Model file for the job. Use its own axes, mm. A direction names the side the tool comes from. Round coordinates to 2 decimals unless told otherwise and drop trailing zeros. Loops run counter-clockwise (first coordinate to the right, second up) from the corner with the lowest first, then second, coordinate; pieces in that order, holes last. Notation, with made-up numbers: M 62,-6 L 100,-6 A24 cw 100,30 Z; hole C 42,68 d3. An arc over 180 degrees is marked long. Answer in a Markdown table with one row per item.
from build123d import *

# Parameters (mm, degrees)
CROQUIS1_R              = 28.9
CROQUIS1_R_2            = 28.6
SALIENTE_EXTRUIR1_DEPTH = 52
CROQUIS2_R              = 17.55
SALIENTE_EXTRUIR2_DEPTH = 52
CROQUIS3_R              = 17.55
CROQUIS3_R_2            = 15
SALIENTE_EXTRUIR3_DEPTH = 2
CROQUIS4_OUTSIDE_W      = 79.374
CROQUIS4_OUTSIDE_H      = 81.026
CROQUIS4_OUTSIDE_R      = 28.9
CORTAR_EXTRUIR1_DEPTH   = 100


with BuildPart() as part:
    # Croquis1 → Saliente-Extruir1 (new body)
    with BuildSketch(Plane(origin=(0, 0, 0), x_dir=(0, 0, -1), z_dir=(1, 0, 0))):
        with Locations(Location((0, 0, 0), (0, 0, 180))):
            Circle(CROQUIS1_R)
        with Locations(Location((0, 0, 0), (0, 0, 180))):
            Circle(CROQUIS1_R_2, mode=Mode.SUBTRACT)
    extrude(amount=SALIENTE_EXTRUIR1_DEPTH)

    # Croquis2 → Saliente-Extruir2 (add)
    with BuildSketch(Plane.ZY):
        with BuildLine():
            Line((-15.676635431, 9.91693509), (-25.360087572, 15.50767879))
            ThreePointArc((-25.360087572, 15.50767879), (-25.743282761, 14.862891232), (-26.110087572, 14.208640684))
            Line((-26.110087572, 14.208640684), (-16.426635431, 8.617896984))
            ThreePointArc((-16.426635431, 8.617896984), (-18.55, 0), (-16.426635431, -8.617896984))
            Line((-16.426635431, -8.617896984), (-26.110087572, -14.208640684))
            ThreePointArc((-26.110087572, -14.208640684), (-25.743282761, -14.862891232), (-25.360087572, -15.50767879))
            Line((-25.360087572, -15.50767879), (-15.676635431, -9.91693509))
            ThreePointArc((-15.676635431, -9.91693509), (-9.275, -16.06477124), (-0.75, -18.534832074))
            Line((-0.75, -18.534832074), (-0.75, -29.716319474))
            ThreePointArc((-0.75, -29.716319474), (0, -29.725782464), (0.75, -29.716319474))
            Line((0.75, -29.716319474), (0.75, -18.534832074))
            ThreePointArc((0.75, -18.534832074), (9.275, -16.06477124), (15.676635431, -9.91693509))
            Line((15.676635431, -9.91693509), (25.360087572, -15.50767879))
            ThreePointArc((25.360087572, -15.50767879), (25.743282761, -14.862891232), (26.110087572, -14.208640684))
            Line((26.110087572, -14.208640684), (16.426635431, -8.617896984))
            ThreePointArc((16.426635431, -8.617896984), (18.55, 0), (16.426635431, 8.617896984))
            Line((16.426635431, 8.617896984), (26.110087572, 14.208640684))
            ThreePointArc((26.110087572, 14.208640684), (25.743282761, 14.862891232), (25.360087572, 15.50767879))
            Line((25.360087572, 15.50767879), (15.676635431, 9.91693509))
            ThreePointArc((15.676635431, 9.91693509), (9.275, 16.06477124), (0.75, 18.534832074))
            Line((0.75, 18.534832074), (0.75, 29.716319474))
            ThreePointArc((0.75, 29.716319474), (0, 29.725782464), (-0.75, 29.716319474))
            Line((-0.75, 29.716319474), (-0.75, 18.534832074))
            ThreePointArc((-0.75, 18.534832074), (-9.275, 16.06477124), (-15.676635431, 9.91693509))
        make_face()
        Circle(CROQUIS2_R, mode=Mode.SUBTRACT)
    extrude(amount=-SALIENTE_EXTRUIR2_DEPTH)

    # Croquis3 → Saliente-Extruir3 (add)
    with BuildSketch(Plane.ZY):
        Circle(CROQUIS3_R)
        Circle(CROQUIS3_R_2, mode=Mode.SUBTRACT)
    extrude(amount=-SALIENTE_EXTRUIR3_DEPTH)

    # Croquis4 outside → Cortar-Extruir1 (cut)
    with BuildSketch(Plane(origin=(52, 0, 0), x_dir=(0, 0, -1), z_dir=(1, 0, 0))):
        Rectangle(CROQUIS4_OUTSIDE_W, CROQUIS4_OUTSIDE_H)
        with Locations(Location((0, 0, 0), (0, 0, 180))):
            Circle(CROQUIS4_OUTSIDE_R, mode=Mode.SUBTRACT)
    extrude(amount=-CORTAR_EXTRUIR1_DEPTH, mode=Mode.SUBTRACT)


solid = part.part
1. Mould opens along Z. For faces 1 (the flat face through (52, 17.3, 4.1)), 2 (the cylindrical face through (25.64, 0.13, -18.55)), 3 (the cylindrical face through (25.636, -20.786, 20.078)) say: +Z half, -Z half, draft (parallel to the pull), parting line (faces both ways), or undercut.
Verdict:
| item | result |
|---|---|
| face 1 | draft |
| face 2 | undercut |
| face 3 | parting line |
2. Saw through at B-B (x = 24). Write the cut outline in (y, z).
Verdict:
| item | result |
|---|---|
| outline | C 0,0 d57.8; hole M -28.59,-0.75 A28.6 ccw -14.94,-24.38 L -9.92,-15.68 A18.55 cw -18.53,-0.75 Z; hole M -28.59,0.75 L -18.53,0.75 A18.55 cw -9.92,15.68 L -14.94,24.38 A28.6 ccw Z; hole C 0,0 d35.1; hole M -13.65,-25.13 A28.6 ccw 13.65,-25.13 L 8.62,-16.43 A18.55 cw -8.62,-16.43 Z; hole M -13.65,25.13 L -8.62,16.43 A18.55 cw 8.62,16.43 L 13.65,25.13 A28.6 ccw Z; hole M 9.92,-15.68 L 14.94,-24.38 A28.6 ccw 28.59,-0.75 L 18.53,-0.75 A18.55 cw Z; hole M 9.92,15.68 A18.55 cw 18.53,0.75 L 28.59,0.75 A28.6 ccw 14.94,24.38 Z |
3. Saw through at C-C (z = 20.5). Write the cut outline in (x, y), and give its area (3 significant figures).
Verdict:
| item | result |
|---|---|
| outline | M 0,-20.37 L 52,-20.37 L 52,-19.94 L 0,-19.94 Z; M 0,-12.7 L 52,-12.7 L 52,-10.97 L 0,-10.97 Z; M 0,10.97 L 52,10.97 L 52,12.7 L 0,12.7 Z; M 0,19.94 L 52,19.94 L 52,20.37 L 0,20.37 Z |
| area | 225 mm² |
4. Saw through at D-D (y = 11). Write the cut outline in (x, z).
Verdict:
| item | result |
|---|---|
| outline | M 0,-26.72 L 52,-26.72 L 52,-26.4 L 0,-26.4 Z; M 0,-20.55 L 52,-20.55 L 52,-17.55 L 0,-17.55 Z; M 0,-14.94 L 52,-14.94 L 52,-13.67 L 2,-13.67 L 2,-10.2 L 0,-10.2 Z; M 0,10.2 L 2,10.2 L 2,13.67 L 52,13.67 L 52,14.94 L 0,14.94 Z; M 0,17.55 L 52,17.55 L 52,20.55 L 0,20.55 Z; M 0,26.4 L 52,26.4 L 52,26.72 L 0,26.72 Z |
5. Wall check: probe 1 along Y at (x, z) = (1, 0); probe 2 along Z at (x, y) = (47.5, 16); probe 3 along Z at (x, y) = (22, 5). Give the ranges that are in metal, low to high.
Verdict:
| item | result |
|---|---|
| probe 1 | y = -28.9 to -15, 15 to 28.9 |
| probe 2 | z = -24.07 to -23.71, -9.39 to -7.21, 7.21 to 9.39, 23.71 to 24.07 |
| probe 3 | z = -28.46 to -28.16, -17.86 to -16.82, 16.82 to 17.86, 28.16 to 28.46 |
6. Tool access for faces 4 (the cylindrical face through (26.65, -10.679, -13.927)), 5 (the flat face through (0, -11, -11)), 6 (the flat face through (25.636, -11.167, 20.842)): list every direction of +Z, -Z, +X, -X, +Y, -Y with a clear straight run to the whole face (end or side of a thin tool).
Verdict:
| item | result |
|---|---|
| face 4 | +X |
| face 5 | +Z, -Z, -X, +Y, -Y |
| face 6 | +X, -X |
7. Pin check, flat tips, straight feed: pin 1 (12 mm diameter, centred on y = 17.5, z = 19.5, fed in from -X); pin 2 (12 mm diameter, centred on x = 30, z = -13, fed in from +Y); pin 3 (5 mm diameter, centred on x = 35.5, y = -23, fed in from +Z); pin 4 (4 mm diameter, centred on y = 8.5, z = 20.5, fed in from +X). Stop position of each tip, or through.
Verdict:
| item | result |
|---|---|
| pin 1 | stops at x = 0 |
| pin 2 | stops at y = 28.04 |
| pin 3 | stops at z = 20.37 |
| pin 4 | passes through |
8. Saw through at A-A (y = 0). Write the cut outline in (x, z).
Verdict:
| item | result |
|---|---|
| outline | M 0,-28.9 L 52,-28.9 L 52,-28.6 L 0,-28.6 Z; M 0,-18.55 L 52,-18.55 L 52,-17.55 L 2,-17.55 L 2,-15 L 0,-15 Z; M 0,15 L 2,15 L 2,17.55 L 52,17.55 L 52,18.55 L 0,18.55 Z; M 0,28.6 L 52,28.6 L 52,28.9 L 0,28.9 Z |
